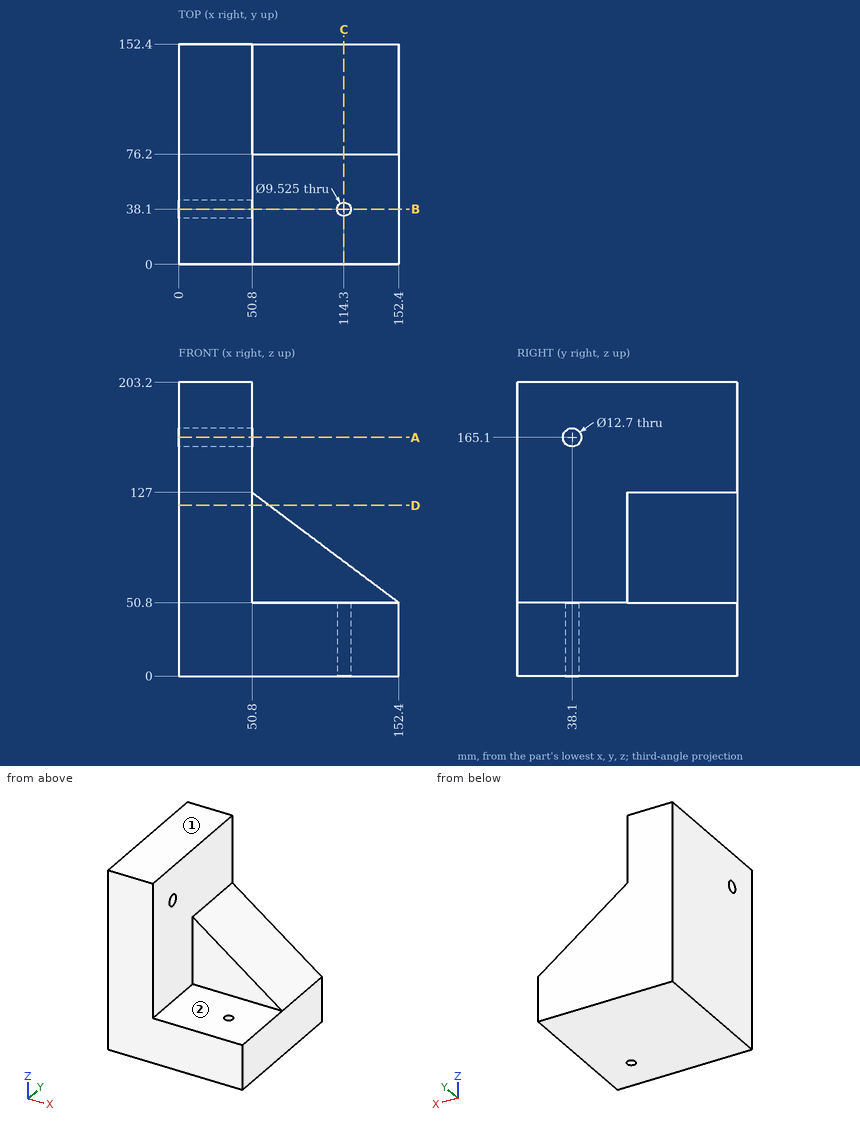
Can you work these out from the drawing? Everything is in mm from the part's minimum corner. A direction names the side the tool comes from. Coordinates: 2 decimals unless noted, no trailing zeros. Loops run counter-clockwise (first coordinate to the right, second up) from the corner with the lowest first, then second, coordinate; pieces in that order, holes last.
1) Which directions (+Z, -Z, +X, -X, +Y, -Y) give clear straight access to the entire face, cutting with the end or side of a thin tool? Please do the marked faces 1 and 2.
Reported:
face 1: +Z, +X, -X, +Y, -Y
face 2: +Z, +X, -Y
2) Imagine slicing it at C-C (x = 114.3). List the corners of the cut face in (y, z) for me (1 decimal), and give its area (3 significant figures).
Reported:
outline: (0, 0) - (33.3, 0) - (33.3, 50.8) - (0, 50.8) - close; (42.9, 0) - (152.4, 0) - (152.4, 79.4) - (76.2, 79.4) - (76.2, 50.8) - (42.9, 50.8) - close
area: 9,440 mm2
3) Please list where these lines run through material, in increasing order: line 1 along Y through (x, z) = (114.3, 11); line 2 along Y through (x, z) = (34, 165); line 3 along X through (y, z) = (57, 185).
Reported:
line 1: y = 0 to 33.34, 42.86 to 152.4
line 2: y = 0 to 31.75, 44.45 to 152.4
line 3: x = 0 to 50.8
4) Imagine slicing it at B-B (y = 38.1). List the corners of the cut face in (x, z) for me.
Reported:
outline: (0, 0) - (109.54, 0) - (109.54, 50.8) - (50.8, 50.8) - (50.8, 158.75) - (0, 158.75) - close; (0, 171.45) - (50.8, 171.45) - (50.8, 203.2) - (0, 203.2) - close; (119.06, 0) - (152.4, 0) - (152.4, 50.8) - (119.06, 50.8) - close
5) Will these pins go through, and if not, where does the flat tip stop? pin 1 Ø11 at (x, y) = (114.3, 38.1) entering from +Z; pin 2 Ø1 at (x, z) = (126, 61.5) entering from -Y; pin 3 Ø20.5 at (y, z) = (38.1, 165.1) entering from +X.
Reported:
pin 1: stops at z = 50.8
pin 2: stops at y = 76.2
pin 3: stops at x = 50.8
6) Imagine slicing it at D-D (z = 118). List the corners of the cut face in (x, y) for me, and give its area (3 significant figures).
Reported:
outline: (0, 0) - (50.8, 0) - (50.8, 76.2) - (62.8, 76.2) - (62.8, 152.4) - (0, 152.4) - close
area: 8,660 mm2
7) Imagine slicing it at A-A (z = 165.1). List the corners of the cut face in (x, y) for me.
Reported:
outline: (0, 0) - (50.8, 0) - (50.8, 31.75) - (0, 31.75) - close; (0, 44.45) - (50.8, 44.45) - (50.8, 152.4) - (0, 152.4) - close
